from build123d import *

# Parameters (mm, degrees)
F0_R     = 1.778
F1_DEPTH = 2.54
F2_R     = 7.5565
F2_R_2   = 5.0165
F3_DEPTH = 6.35
F4_R     = 5.08
F5_R     = 1.016
F6_R     = 1.778
F7_DEPTH = 25.4


with BuildPart() as f1:
    # F0 (on Front) → F1 (new body)
    with BuildSketch(Plane.XZ):
        with BuildLine():
            ThreePointArc((7.605604, -0.468175), (7.6164, -0.234198), (7.62, 0))
            ThreePointArc((7.62, 0), (7.6164, 0.234198), (7.605604, 0.468175))
            ThreePointArc((7.605604, 0.468175), (7.247051, 2.354709), (6.428249, 4.0917))
            ThreePointArc((6.428249, 4.0917), (6.164709, 4.478924), (5.877877, 4.849223))
            ThreePointArc((5.877877, 4.849223), (4.478924, 6.164709), (2.795522, 7.088685))
            ThreePointArc((2.795522, 7.088685), (2.354709, 7.247051), (1.905, 7.378033))
            ThreePointArc((1.905, 7.378033), (0, 7.62), (-1.905, 7.378033))
            ThreePointArc((-1.905, 7.378033), (-2.354709, 7.247051), (-2.795522, 7.088685))
            ThreePointArc((-2.795522, 7.088685), (-4.478924, 6.164709), (-5.877877, 4.849223))
            ThreePointArc((-5.877877, 4.849223), (-6.164709, 4.478924), (-6.428249, 4.0917))
            ThreePointArc((-6.428249, 4.0917), (-7.247051, 2.354709), (-7.605604, 0.468175))
            ThreePointArc((-7.605604, 0.468175), (-7.62, 0), (-7.605604, -0.468175))
            ThreePointArc((-7.605604, -0.468175), (-7.247051, -2.354709), (-6.428249, -4.0917))
            ThreePointArc((-6.428249, -4.0917), (-6.164709, -4.478924), (-5.877877, -4.849223))
            ThreePointArc((-5.877877, -4.849223), (-4.478924, -6.164709), (-2.795522, -7.088685))
            ThreePointArc((-2.795522, -7.088685), (-2.354709, -7.247051), (-1.905, -7.378033))
            ThreePointArc((-1.905, -7.378033), (0, -7.62), (1.905, -7.378033))
            ThreePointArc((1.905, -7.378033), (2.354709, -7.247051), (2.795522, -7.088685))
            ThreePointArc((2.795522, -7.088685), (4.478924, -6.164709), (5.877877, -4.849223))
            ThreePointArc((5.877877, -4.849223), (6.164709, -4.478924), (6.428249, -4.0917))
            ThreePointArc((6.428249, -4.0917), (7.247051, -2.354709), (7.605604, -0.468175))
        make_face()
        Circle(F0_R, mode=Mode.SUBTRACT)
        with BuildLine():
            ThreePointArc((6.428249, 4.0917), (7.247051, 2.354709), (7.605604, 0.468175))
            Line((7.605604, 0.468175), (9.689785, 1.412438))
            Line((9.689785, 1.412438), (11.830752, 3.04283))
            Line((11.830752, 3.04283), (11.35981, 4.49224))
            Line((11.35981, 4.49224), (8.66941, 4.552826))
            Line((8.66941, 4.552826), (6.428249, 4.0917))
        make_face()
        with BuildLine():
            Line((9.689785, -1.412438), (7.605604, -0.468175))
            ThreePointArc((7.605604, -0.468175), (7.247051, -2.354709), (6.428249, -4.0917))
            Line((6.428249, -4.0917), (8.66941, -4.552826))
            Line((8.66941, -4.552826), (11.35981, -4.49224))
            Line((11.35981, -4.49224), (11.830752, -3.04283))
            Line((11.830752, -3.04283), (9.689785, -1.412438))
        make_face()
        with BuildLine():
            ThreePointArc((2.795522, 7.088685), (4.478924, 6.164709), (5.877877, 4.849223))
            Line((5.877877, 4.849223), (7.00899, 6.838199))
            Line((7.00899, 6.838199), (7.782749, 9.415643))
            Line((7.782749, 9.415643), (6.549807, 10.311428))
            Line((6.549807, 10.311428), (4.337616, 8.779065))
            Line((4.337616, 8.779065), (2.795522, 7.088685))
        make_face()
        with BuildLine():
            Line((7.00899, -6.838199), (5.877877, -4.849223))
            ThreePointArc((5.877877, -4.849223), (4.478924, -6.164709), (2.795522, -7.088685))
            Line((2.795522, -7.088685), (4.337616, -8.779065))
            Line((4.337616, -8.779065), (6.549807, -10.311428))
            Line((6.549807, -10.311428), (7.782749, -9.415643))
            Line((7.782749, -9.415643), (7.00899, -6.838199))
        make_face()
        with BuildLine():
            ThreePointArc((-1.905, 7.378033), (0, 7.62), (1.905, 7.378033))
            Line((1.905, 7.378033), (1.651, 9.652))
            Line((1.651, 9.652), (0.762, 12.192))
            Line((0.762, 12.192), (-0.762, 12.192))
            Line((-0.762, 12.192), (-1.651, 9.652))
            Line((-1.651, 9.652), (-1.905, 7.378033))
        make_face()
        with BuildLine():
            Line((1.651, -9.652), (1.905, -7.378033))
            ThreePointArc((1.905, -7.378033), (0, -7.62), (-1.905, -7.378033))
            Line((-1.905, -7.378033), (-1.651, -9.652))
            Line((-1.651, -9.652), (-0.762, -12.192))
            Line((-0.762, -12.192), (0.762, -12.192))
            Line((0.762, -12.192), (1.651, -9.652))
        make_face()
        with BuildLine():
            ThreePointArc((-5.877877, 4.849223), (-4.478924, 6.164709), (-2.795522, 7.088685))
            Line((-2.795522, 7.088685), (-4.337616, 8.779065))
            Line((-4.337616, 8.779065), (-6.549807, 10.311428))
            Line((-6.549807, 10.311428), (-7.782749, 9.415643))
            Line((-7.782749, 9.415643), (-7.00899, 6.838199))
            Line((-7.00899, 6.838199), (-5.877877, 4.849223))
        make_face()
        with BuildLine():
            Line((-4.337616, -8.779065), (-2.795522, -7.088685))
            ThreePointArc((-2.795522, -7.088685), (-4.478924, -6.164709), (-5.877877, -4.849223))
            Line((-5.877877, -4.849223), (-7.00899, -6.838199))
            Line((-7.00899, -6.838199), (-7.782749, -9.415643))
            Line((-7.782749, -9.415643), (-6.549807, -10.311428))
            Line((-6.549807, -10.311428), (-4.337616, -8.779065))
        make_face()
        with BuildLine():
            ThreePointArc((-7.605604, 0.468175), (-7.247051, 2.354709), (-6.428249, 4.0917))
            Line((-6.428249, 4.0917), (-8.66941, 4.552826))
            Line((-8.66941, 4.552826), (-11.35981, 4.49224))
            Line((-11.35981, 4.49224), (-11.830752, 3.04283))
            Line((-11.830752, 3.04283), (-9.689785, 1.412438))
            Line((-9.689785, 1.412438), (-7.605604, 0.468175))
        make_face()
        with BuildLine():
            Line((-8.66941, -4.552826), (-6.428249, -4.0917))
            ThreePointArc((-6.428249, -4.0917), (-7.247051, -2.354709), (-7.605604, -0.468175))
            Line((-7.605604, -0.468175), (-9.689785, -1.412438))
            Line((-9.689785, -1.412438), (-11.830752, -3.04283))
            Line((-11.830752, -3.04283), (-11.35981, -4.49224))
            Line((-11.35981, -4.49224), (-8.66941, -4.552826))
        make_face()
    extrude(amount=F1_DEPTH)

    # F2 (on face) → F3 (join)
    with BuildSketch(Plane.XZ.offset(2.54)):
        Circle(F2_R)
        Circle(F2_R_2, mode=Mode.SUBTRACT)
    extrude(amount=F3_DEPTH)

    # F4
    f4_edges = [f1.edges().sort_by_distance(p)[0] for p in [
        (7.00899, -1.27, 6.838199),
        (4.337616, -1.27, 8.779065),
        (1.651, -1.27, 9.652),
        (-4.337616, -1.27, 8.779065),
        (-8.66941, -1.27, 4.552826),
        (-9.689785, -1.27, -1.412438),
        (-7.00899, -1.27, -6.838199),
        (-1.651, -1.27, -9.652),
        (4.337616, -1.27, -8.779065),
        (8.66941, -1.27, -4.552826),
        (9.689785, -1.27, 1.412438),
        (9.689785, -1.27, -1.412438),
        (8.66941, -1.27, 4.552826),
        (-1.651, -1.27, 9.652),
        (-7.00899, -1.27, 6.838199),
        (-9.689785, -1.27, 1.412438),
        (-8.66941, -1.27, -4.552826),
        (-4.337616, -1.27, -8.779065),
        (1.651, -1.27, -9.652),
        (7.00899, -1.27, -6.838199),
    ]]
    fillet(f4_edges, radius=F4_R)

    # F5
    f5_edges = [f1.edges().sort_by_distance(p)[0] for p in [
        (0.762, -1.27, 12.192),
        (-0.762, -1.27, 12.192),
        (-6.549807, -1.27, 10.311428),
        (-7.782749, -1.27, 9.415643),
        (-11.35981, -1.27, 4.49224),
        (6.549807, -1.27, 10.311428),
        (7.782749, -1.27, 9.415643),
        (11.35981, -1.27, 4.49224),
        (-11.830752, -1.27, 3.04283),
        (-11.830752, -1.27, -3.04283),
        (-11.35981, -1.27, -4.49224),
        (-7.782749, -1.27, -9.415643),
        (-6.549807, -1.27, -10.311428),
        (-0.762, -1.27, -12.192),
        (0.762, -1.27, -12.192),
        (6.549807, -1.27, -10.311428),
        (7.782749, -1.27, -9.415643),
        (11.830752, -1.27, -3.04283),
        (11.35981, -1.27, -4.49224),
        (11.830752, -1.27, 3.04283),
    ]]
    fillet(f5_edges, radius=F5_R)

    # F6 (on Top) → F7 (cut)
    with BuildSketch(Plane.XY):
        with Locations((0, -5.461)):
            Circle(F6_R)
    extrude(amount=F7_DEPTH, mode=Mode.SUBTRACT)


solid = f1.part
Can you work these out from the model? Positions are in its coordinate system, mm. A direction names the side the tool comes from. Give positions to 0.01 mm unless a question says otherwise; leave off trailing zeros. Loops run counter-clockwise (first coordinate to the right, second up) from the corner with the lowest first, then second, coordinate; pieces in that order, holes last. Notation, with made-up numbers: M 84,48 L 105,48 A34 cw 105,87 Z; hole C 61.25,10.25 d4. An arc over 180 degrees is marked long. One line per item, written item: value.
1) Imagine slicing it at B-B on y = -3. Write out the boundary of the cut face in (x, z).
Geometry check:
outline: C 0,0 d15.11; hole C 0,0 d10.03
2) Please list where these lines run through material, in increasing order: line 1 (Z direction, x = 0, y = -1.05); line 2 (Y direction, x = 0, z = 5.65); line 3 (X direction, y = -0.5, z = 9.5).
Geometry check:
line 1: z = -12.19 to -1.78, 1.78 to 12.19
line 2: y = -8.89 to -7.24, -3.68 to 0
line 3: x = -7.5 to -5.38, -1.65 to 1.65, 5.38 to 7.5
3) I'm going to push flat-ended pins straight in: pin 1 (2 mm diameter, centred on x = 1, z = 1, fed in from -Y); pin 2 (3 mm diameter, centred on x = 0, y = -5.461, fed in from -Z); pin 3 (3 mm diameter, centred on y = -5.5, z = -3.5, fed in from -X). Where does each tip first touch, or does it pass through?
Geometry check:
pin 1: stops at y = -2.54
pin 2: stops at z = -7.56
pin 3: stops at x = -7.29
4) On a 3-axis mill with a long thin cutter (end or side, diameter ignored), from which of +Z, -Z, +X, -X, +Y, -Y can I reach the whole of each face in a straight line? I mean faces 4 (the face through (8.4, -1.25, -0.83)), 5 (the face through (-8.66, -1.29, 4.52)), 6 (the face through (-7.255, -1.252, 4.262)), 7 (the face through (1.62, -1.29, -9.65)), 8 (the face through (-11.22, -1.29, -4.31)). Say none if no direction works.
Geometry check:
face 4: +X, +Y, -Y
face 5: +Z, +Y, -Y
face 6: +Y, -Y
face 7: -Z, +Y, -Y
face 8: -Z, -X, +Y, -Y
5) Imagine slicing it at A-A on z = 6. Write out the boundary of the cut face in (x, y), and give its area (3 significant figures).
Geometry check:
outline: M -6.53,-2.54 L -4.59,-2.54 L -4.59,-8.89 L 4.59,-8.89 L 4.59,-2.54 L 6.53,-2.54 L 6.53,0 L -6.53,0 Z; hole C 0,-5.46 d3.56
area: 81.6 mm²
6) Imagine slicing it at C-C on x = -3.25. Write out the boundary of the cut face in (y, z).
Geometry check:
outline: M -8.89,-6.82 L -2.54,-6.82 L -2.54,-7.59 L 0,-7.59 L 0,7.59 L -2.54,7.59 L -2.54,6.82 L -8.89,6.82 L -8.89,3.82 L -2.54,3.82 L -2.54,-3.82 L -8.89,-3.82 Z
7) Imagine slicing it at D-D on z = 10.5. Write out the boundary of the cut face in (x, y).
Geometry check:
outline: M -1.35,-2.54 L 1.35,-2.54 L 1.35,0 L -1.35,0 Z
8) Thinking about a two-plate mould opening in X: for faces 1 (the face through (7.57, -1.29, 9.33)), 2 (the face through (-1.234, -1.252, -10.844)), 3 (the face through (-1.62, -1.29, 9.65)), which applies, +X half, -X half, draft (parallel to the pull), parting line (faces both ways), or undercut?
Geometry check:
face 1: +X half
face 2: -X half
face 3: undercut
